Read the model definition and answer for the solid it produces. Units are mm, in the model's axes. Face numbers are marked on the shaded views. A direction names the side the tool comes from. Give positions to 0.01 mm unless a question says otherwise; leave off trailing zeros. Order: outer loops, then holes, each group sorted by start corner. A loop starts at its lowest first (then second) coordinate and runs counter-clockwise, first axis right, second up. Notation, with made-up numbers: (-7, 27) - (44, 27) arc R37 cw to (44, 65) - close; hole circle Ø5 at (-26, 54.5). An arc over 180 degrees is marked (long way). Write each question's results on one line, items separated by ' | '. Start each with the question number.
Q1. Find section B-B on x = 5. Give the vertices of the cut face in (y, z).
Q2. Find section D-D on y = 0.35. Give the vertices of the cut face in (x, z).
Q3. Flat-ended cylindrical pins translate along their axes: P1, Ø1.5, axis at x = 3.5, y = 1.5, coming from the -Z side; P2, Ø3, axis at x = 7, z = 13, coming from the +Y side; P3, Ø1, axis at x = 3, y = 3, coming from the +Z side. Find the tip coordinate at first contact, or state that the pin passes through.
Q4. Find section C-C on y = 2.4. Give the vertices of the cut face in (x, z).
Q5. Find the intervals of material crossed by line 1 along X through (y, z) = (0.55, 12.35); line 2 along Z through (x, y) = (5, 4.3); line 3 along Y through (x, z) = (8.5, 12.5), in increasing order. Write a range as from..to.
Q6. Find section A-A on z = 12.35. Give the vertices of the cut face in (x, y).
Q7. A tool of negligible diameter and unlimited length cuts with its end or side. For the marked faces 1 and 2, from which of +Z, -Z, +X, -X, +Y, -Y can it reach the whole face along a straight path? Write none if from no direction.
from build123d import *

# Parameters (mm, degrees)
SKETCH_1_W          = 10
SKETCH_1_H          = 4.4
EXTRUDE_1_DEPTH     = 15.2
SKETCH_2_W          = 6.2
SKETCH_2_H          = 3.2
CUT_EXTRUDE_1_DEPTH = 19.718974331
CUT_EXTRUDE_2_REACH = 20.719
SKETCH_3_R          = 1.85
SKETCH_4_R          = 0.816532351
CUT_EXTRUDE_3_DEPTH = 0.2
EXTRUDE_2_DEPTH     = 2
WRAP_START          = -0.2
WRAP_1_DEPTH        = 0.2


# Read off the part's stored shape, not the designer's step: 包覆1
with BuildPart() as part:
    # 草图1 → 凸台-拉伸1 (new body)
    with BuildSketch(Plane.XY):
        with Locations((5, 2.2)):
            Rectangle(SKETCH_1_W, SKETCH_1_H)
    extrude(amount=EXTRUDE_1_DEPTH)

    # 草图2 → 切除-拉伸1 (cut, through all)
    with BuildSketch(Plane(origin=(10, 0, 0), x_dir=(0, 0, -1), z_dir=(1, 0, 0))):
        with Locations((-12.1, 2.8)):
            Rectangle(SKETCH_2_W, SKETCH_2_H)
    extrude(amount=-CUT_EXTRUDE_1_DEPTH, mode=Mode.SUBTRACT)

    # 草图3 → 切除-拉伸2 (cut, up to next)
    with BuildSketch(Plane.XZ, mode=Mode.PRIVATE) as cut_extrude_2_sk1:
        with Locations(Location((5, 12.35, 0), (0, 0, 270))):
            Circle(SKETCH_3_R)
    cut_extrude_2_tool1 = extrude(cut_extrude_2_sk1.sketch, amount=-CUT_EXTRUDE_2_REACH, mode=Mode.PRIVATE) & part.part
    add(cut_extrude_2_tool1.solids().sort_by_distance((5, 0, 12.35))[0], mode=Mode.SUBTRACT)

    # 草图4 → 切除-拉伸3 (cut)
    with BuildSketch(Plane(origin=(0, 4.4, 0), x_dir=(-1, 0, 0), z_dir=(0, 1, 0))):
        with Locations((-5, 7.32228291)):
            Circle(SKETCH_4_R)
    extrude(amount=-CUT_EXTRUDE_3_DEPTH, mode=Mode.SUBTRACT)

    # 草图5 → 凸台-拉伸2 (add)
    with BuildSketch(Plane(origin=(0, 0, 0), x_dir=(-1, 0, 0), z_dir=(0, 0, -1))):
        with BuildLine():
            Line((-7.94, 2.65), (-7.14, 2.65))
            ThreePointArc((-7.14, 2.65), (-6.89, 2.4), (-7.14, 2.15))
            Line((-7.14, 2.15), (-7.94, 2.15))
            ThreePointArc((-7.94, 2.15), (-8.19, 2.4), (-7.94, 2.65))
        make_face()
        with BuildLine():
            Line((-2.06, 2.65), (-2.86, 2.65))
            ThreePointArc((-2.86, 2.65), (-3.11, 2.4), (-2.86, 2.15))
            Line((-2.86, 2.15), (-2.06, 2.15))
            ThreePointArc((-2.06, 2.15), (-1.81, 2.4), (-2.06, 2.65))
        make_face()
    extrude(amount=EXTRUDE_2_DEPTH)

    # 包覆1 outline → 包覆1 (cut)
    # profile 1 of 2: a face of its own
    with BuildSketch(Plane(origin=(0, 4.4, 0), x_dir=(1, 0, 0), z_dir=(0, 1, 0)).offset(WRAP_START)):
        with BuildLine():
            add(Edge.make_bspline(
                [(6.930989583, -2.031758229), (6.915107326, -2.032625879), (6.886212727, -2.034204394), (6.846667333, -2.045372179), (6.819228063, -2.069428088), (6.803221049, -2.101586149), (6.801017387, -2.141193863), (6.810949266, -2.186053613), (6.830123901, -2.237549844), (6.849896632, -2.272058221), (6.860677083, -2.290872813)],
                knots=[0, 0, 0, 0, 0.134063604, 0.243901978, 0.338487503, 0.432506005, 0.538929196, 0.665491452, 0.817619881, 1, 1, 1, 1], degree=3))
            Line((6.930989583, -2.031758229), (6.983723958, -2.031758229))
            Line((6.983723958, -2.031758229), (6.983723958, -1.906758229))
            Line((6.983723958, -1.906758229), (6.208333333, -1.906758229))
            Line((6.208333333, -1.906758229), (6.208333333, -2.031758229))
            Line((6.208333333, -2.031758229), (6.295572917, -2.031758229))
            add(Edge.make_bspline(
                [(6.504557292, -2.221862396), (6.495929833, -2.205652704), (6.479665398, -2.175094288), (6.45244636, -2.133930793), (6.422954526, -2.101143884), (6.393052529, -2.075772209), (6.364287696, -2.056836396), (6.33849766, -2.04342026), (6.316216749, -2.033596626), (6.301937753, -2.032325038), (6.295572917, -2.031758229)],
                knots=[0, 0, 0, 0, 0.187742948, 0.353931892, 0.503213882, 0.637048905, 0.753995091, 0.854253228, 0.93503364, 1, 1, 1, 1], degree=3))
            Line((6.504557292, -2.221862396), (7.255859375, -3.800638438))
            Line((7.255859375, -3.800638438), (6.711588542, -4.574075938))
            add(Edge.make_bspline(
                [(6.367838542, -4.781758229), (6.382221439, -4.781136361), (6.411311872, -4.779878589), (6.454540631, -4.769294334), (6.498129706, -4.753858707), (6.541134976, -4.730459287), (6.584266179, -4.700950899), (6.627240555, -4.66479857), (6.670366285, -4.622362568), (6.697506142, -4.590571678), (6.711588542, -4.574075938)],
                knots=[0, 0, 0, 0, 0.103884895, 0.210114587, 0.320338877, 0.43759129, 0.56296606, 0.6978075, 0.843197564, 1, 1, 1, 1], degree=3))
            Line((6.367838542, -4.781758229), (6.333333333, -4.781758229))
            Line((6.333333333, -4.781758229), (6.333333333, -4.906758229))
            Line((6.333333333, -4.906758229), (7.063802083, -4.906758229))
            Line((7.063802083, -4.906758229), (7.063802083, -4.781758229))
            Line((7.063802083, -4.781758229), (6.993489583, -4.781758229))
            add(Edge.make_bspline(
                [(6.888020833, -4.539570729), (6.875914449, -4.558101633), (6.854053882, -4.591562992), (6.832516724, -4.641371555), (6.825349297, -4.68501694), (6.834657735, -4.72263487), (6.859636327, -4.75025169), (6.89505428, -4.769644136), (6.941090575, -4.779777335), (6.974999933, -4.781059246), (6.993489583, -4.781758229)],
                knots=[0, 0, 0, 0, 0.178363102, 0.322071271, 0.434997506, 0.529283499, 0.62366698, 0.72638665, 0.850807703, 1, 1, 1, 1], degree=3))
            Line((6.888020833, -4.539570729), (7.708333333, -3.374206146))
            Line((7.708333333, -3.374206146), (7.708333333, -4.642435313))
            add(Edge.make_bspline(
                [(7.55859375, -4.781758229), (7.569261505, -4.781466132), (7.589734391, -4.780905556), (7.618905697, -4.774334821), (7.644615767, -4.763072355), (7.667304115, -4.748054599), (7.686035697, -4.728256372), (7.69919622, -4.703300066), (7.707027639, -4.674151855), (7.707884523, -4.653337332), (7.708333333, -4.642435313)],
                knots=[0, 0, 0, 0, 0.137639342, 0.264148789, 0.383430361, 0.498519415, 0.613574313, 0.731497168, 0.859366305, 1, 1, 1, 1], degree=3))
            Line((7.55859375, -4.781758229), (7.458333333, -4.781758229))
            Line((7.458333333, -4.781758229), (7.458333333, -4.906758229))
            Line((7.458333333, -4.906758229), (8.25, -4.906758229))
            Line((8.25, -4.906758229), (8.25, -4.781758229))
            Line((8.25, -4.781758229), (8.149739583, -4.781758229))
            add(Edge.make_bspline(
                [(8, -4.643086354), (8.000247716, -4.65398027), (8.000713759, -4.674475698), (8.007493922, -4.70308304), (8.017717416, -4.727550741), (8.032366625, -4.748243586), (8.05327597, -4.763833527), (8.080059672, -4.774757464), (8.113000414, -4.780982371), (8.136907743, -4.781487246), (8.149739583, -4.781758229)],
                knots=[0, 0, 0, 0, 0.137957594, 0.25954853, 0.370573832, 0.47303595, 0.577150492, 0.696855208, 0.837292342, 1, 1, 1, 1], degree=3))
            Line((8, -4.643086354), (8, -2.170430104))
            add(Edge.make_bspline(
                [(8.149739583, -2.031758229), (8.136907977, -2.032029309), (8.113001084, -2.032534363), (8.080057551, -2.038758127), (8.053282295, -2.049685522), (8.032346439, -2.065264608), (8.017909992, -2.085832582), (8.007221233, -2.110117779), (8.000820991, -2.138857995), (8.00028302, -2.159546252), (8, -2.170430104)],
                knots=[0, 0, 0, 0, 0.162681349, 0.303095774, 0.422781134, 0.526878841, 0.629324391, 0.737809695, 0.862064713, 1, 1, 1, 1], degree=3))
            Line((8.149739583, -2.031758229), (8.25, -2.031758229))
            Line((8.25, -2.031758229), (8.25, -1.906758229))
            Line((8.25, -1.906758229), (7.458333333, -1.906758229))
            Line((7.458333333, -1.906758229), (7.458333333, -2.031758229))
            Line((7.458333333, -2.031758229), (7.55859375, -2.031758229))
            add(Edge.make_bspline(
                [(7.708333333, -2.170430104), (7.707872164, -2.159534741), (7.706991684, -2.138732927), (7.699369622, -2.109684264), (7.685819191, -2.085165103), (7.667326615, -2.065449868), (7.644609508, -2.05044744), (7.618907501, -2.039180676), (7.589733882, -2.032611175), (7.569261331, -2.03205042), (7.55859375, -2.031758229)],
                knots=[0, 0, 0, 0, 0.14098033, 0.269164641, 0.384913342, 0.500251829, 0.615624556, 0.735200135, 0.862021403, 1, 1, 1, 1], degree=3))
            Line((7.708333333, -2.170430104), (7.708333333, -3.156107188))
            Line((7.708333333, -3.156107188), (7.448567708, -3.525898854))
            Line((7.448567708, -3.525898854), (6.860677083, -2.290872813))
        make_face()
    # profile 2 of 2: a face of its own
    with BuildSketch(Plane(origin=(0, 4.4, 0), x_dir=(1, 0, 0), z_dir=(0, 1, 0)).offset(WRAP_START)):
        with BuildLine():
            add(Edge.make_bspline(
                [(3.418619792, -2.355325938), (3.423290626, -2.332189778), (3.432052726, -2.288788256), (3.436281258, -2.225966665), (3.432219716, -2.170311627), (3.419748545, -2.121523718), (3.397043855, -2.080672541), (3.361471203, -2.050596509), (3.313901494, -2.03475832), (3.27919164, -2.032811362), (3.260416667, -2.031758229)],
                knots=[0, 0, 0, 0, 0.164440403, 0.308476601, 0.437530233, 0.552061218, 0.657168364, 0.758108431, 0.86915797, 1, 1, 1, 1], degree=3))
            Line((3.418619792, -2.355325938), (3.251302083, -3.031758229))
            Line((3.251302083, -3.031758229), (2.47265625, -3.031758229))
            Line((2.47265625, -3.031758229), (2.284505208, -2.243346771))
            add(Edge.make_bspline(
                [(2.407552083, -2.031758229), (2.391667135, -2.032296875), (2.362566209, -2.033283664), (2.3231508, -2.042204366), (2.293092672, -2.059473632), (2.273233438, -2.084737484), (2.26487379, -2.11648377), (2.262976163, -2.153509682), (2.270537673, -2.196694946), (2.279598478, -2.226958202), (2.284505208, -2.243346771)],
                knots=[0, 0, 0, 0, 0.152863017, 0.280042176, 0.385019123, 0.480297622, 0.580749292, 0.695821655, 0.835277215, 1, 1, 1, 1], degree=3))
            Line((2.407552083, -2.031758229), (2.477864583, -2.031758229))
            Line((2.477864583, -2.031758229), (2.477864583, -1.906758229))
            Line((2.477864583, -1.906758229), (1.708333333, -1.906758229))
            Line((1.708333333, -1.906758229), (1.708333333, -2.031758229))
            Line((1.708333333, -2.031758229), (1.761067708, -2.031758229))
            add(Edge.make_bspline(
                [(1.972005208, -2.192565521), (1.966073989, -2.178707602), (1.9549211, -2.152649581), (1.933551487, -2.118325589), (1.911064572, -2.089505922), (1.884961055, -2.067865098), (1.857221348, -2.050878644), (1.826723244, -2.040325548), (1.794671237, -2.032437792), (1.772404332, -2.031987489), (1.761067708, -2.031758229)],
                knots=[0, 0, 0, 0, 0.158644365, 0.298310162, 0.425134921, 0.541996665, 0.653801398, 0.765979904, 0.880854674, 1, 1, 1, 1], degree=3))
            Line((1.972005208, -2.192565521), (2.639322917, -4.990091563))
            Line((2.639322917, -4.990091563), (2.918619792, -4.902851979))
            Line((2.918619792, -4.902851979), (3.587239583, -2.224466563))
            add(Edge.make_bspline(
                [(3.780598958, -2.031758229), (3.769253734, -2.032178513), (3.74688055, -2.033007326), (3.714560239, -2.042036162), (3.684338324, -2.05569344), (3.656371612, -2.074852871), (3.631282534, -2.10088588), (3.612447742, -2.135739762), (3.596389822, -2.177235982), (3.590420449, -2.208047958), (3.587239583, -2.224466563)],
                knots=[0, 0, 0, 0, 0.1127485, 0.22234404, 0.331662042, 0.442001332, 0.558219825, 0.688003095, 0.833747961, 1, 1, 1, 1], degree=3))
            Line((3.780598958, -2.031758229), (3.833333333, -2.031758229))
            Line((3.833333333, -2.031758229), (3.833333333, -1.906758229))
            Line((3.833333333, -1.906758229), (3.207682292, -1.906758229))
            Line((3.207682292, -1.906758229), (3.207682292, -2.031758229))
            Line((3.207682292, -2.031758229), (3.260416667, -2.031758229))
        make_face()
        Polygon((2.485026042, -3.156758229), (3.221354167, -3.156758229), (2.861979167, -4.612487396), (2.829427083, -4.604674896), align=None, mode=Mode.SUBTRACT)
    extrude(amount=WRAP_1_DEPTH, mode=Mode.SUBTRACT)


solid = part.part
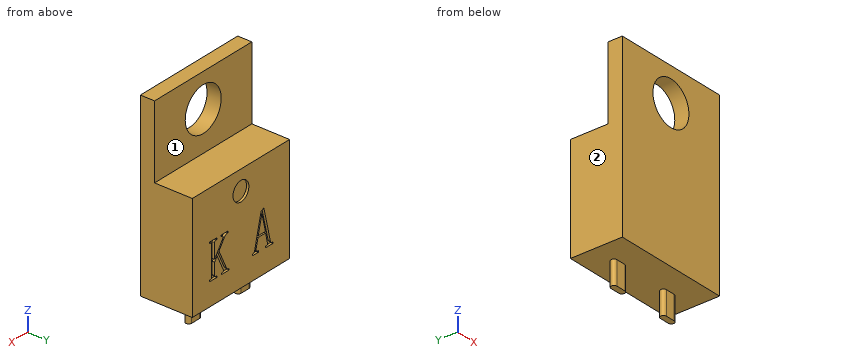
Working result:
1) outline: (0, 0) - (4.4, 0) - (4.4, 6.51) - (4.2, 6.51) - (4.2, 8.14) - (4.4, 8.14) - (4.4, 9) - (1.2, 9) - (1.2, 10.5) - (0, 10.5) - close; (0, 14.2) - (1.2, 14.2) - (1.2, 15.2) - (0, 15.2) - close
2) outline: (0, 0) - (10, 0) - (10, 15.2) - (0, 15.2) - close; hole circle Ø3.7 at (5, 12.35)
3) P1: z = 0 | P2: y = 1.2 | P3: z = 9
4) outline: (0, 0) - (1.81, 0) - (1.81, -2) - (3.11, -2) - (3.11, 0) - (6.89, 0) - (6.89, -2) - (8.19, -2) - (8.19, 0) - (10, 0) - (10, 9) - (0, 9) - close
5) line 1: 0..3.15, 6.85..10 | line 2: 0..6.51, 8.14..9 | line 3: 0..1.2
6) outline: (0, 0) - (3.15, 0) - (3.15, 1.2) - (0, 1.2) - close; (6.85, 0) - (10, 0) - (10, 1.2) - (6.85, 1.2) - close
7) face 1: +Z, +X, -X, +Y | face 2: +Z, -Z, -X, +Y, -Y
